```python
from build123d import *

# Parameters (mm, degrees)
F0_W        = 33.02
F0_H        = 101.6
F1_DEPTH    = 2.54
F2_W        = 33.02
F2_H        = 101.6
F2_W_2      = 5.08
F2_H_2      = 2.54
F3_DEPTH    = 19.05
F2_W_3      = 27.94
F2_H_3      = 27.94
F2_W_4      = 1.8288
F2_H_4      = 4.572
F4_DEPTH    = 2.54
F5_DEPTH    = 5.08
F7_W        = 3.1588217151
F7_H        = 3.175
F8_DEPTH    = 25.4
F9_T1_DEPTH = 2.54
F10_W       = 0.4572
F10_H       = 4.572
F10_W_2     = 1.8288
F10_W_3     = 2.286
F11_DEPTH   = 1.27
F13_DEPTH   = 6.35


# Not quite as in the source:
# - a fillet or chamfer that OpenCascade refuses, or shapes differently, is made with other operations: its cross-section is extruded or revolved along the edge and cut away or added


with BuildPart() as f1:
    # F0 (on Top) → F1 (new body)
    with BuildSketch(Plane.XY):
        with Locations((16.51, 50.8)):
            Rectangle(F0_W, F0_H)
    extrude(amount=F1_DEPTH)

    # F2 (on face) → F3 (join)
    with BuildSketch(Plane.XY.offset(2.54)):
        with Locations((16.51, 50.8)):
            Rectangle(F2_W, F2_H)
        Polygon((30.48, 2.54), (2.54, 2.54), (2.54, 64.77), (2.54, 67.31), (2.54, 71.12), (2.54, 99.06), (30.48, 99.06), (30.48, 71.12), (30.48, 67.31), (30.48, 64.77), align=None, mode=Mode.SUBTRACT)
        with Locations((5.08, 66.04)):
            Rectangle(F2_W_2, F2_H_2)
        with Locations((27.94, 66.04)):
            Rectangle(F2_W_2, F2_H_2)
    extrude(amount=F3_DEPTH)

    # F2 (on face) → F4 (join)
    with BuildSketch(Plane.XY.offset(2.54)):
        with Locations((16.51, 85.09)):
            Rectangle(F2_W_3, F2_H_3)
        with Locations((9.8806, 82.3468)):
            Rectangle(F2_W_4, F2_H_4, mode=Mode.SUBTRACT)
        with Locations((23.1394, 82.3468)):
            Rectangle(F2_W_4, F2_H_4, mode=Mode.SUBTRACT)
    extrude(amount=F4_DEPTH)

    # F2 (on face) → F5 (join)
    with BuildSketch(Plane.XY.offset(2.54)):
        with Locations((9.8806, 82.3468)):
            Rectangle(F2_W_4, F2_H_4)
        with Locations((23.1394, 82.3468)):
            Rectangle(F2_W_4, F2_H_4)
    extrude(amount=F5_DEPTH)

    # F7 (on face) → F8 (cut)
    with BuildSketch(Plane.XZ.offset(-99.06)):
        Polygon((10.795, 9.525), (10.795, 8.89), (24.0538, 8.89), (24.0538, 21.59), (10.795, 21.59), (10.795, 12.7), align=None)
        with Locations((9.2155891424, 11.1125)):
            Rectangle(F7_W, F7_H)
    extrude(amount=-F8_DEPTH, mode=Mode.SUBTRACT)

    # F9: fillet of radius 1.651 on 2 edges, made by hand

    # F9_s2 → F9_t1 (join)
    with BuildSketch(Plane.XZ.offset(-101.6)):
        with BuildLine():
            ThreePointArc((9.2871782849, 12.7), (8.1197449891, 12.2164332957), (7.6361782849, 11.049))
            Line((7.6361782849, 11.049), (7.6361782849, 12.7))
            Line((7.6361782849, 12.7), (9.2871782849, 12.7))
        make_face()
        with BuildLine():
            ThreePointArc((7.6361782849, 11.176), (8.1197449891, 10.0085667043), (9.2871782849, 9.525))
            Line((9.2871782849, 9.525), (7.6361782849, 9.525))
            Line((7.6361782849, 9.525), (7.6361782849, 11.176))
        make_face()
    extrude(amount=F9_T1_DEPTH)

    # F10 (on face) → F11 (join)
    with BuildSketch(Plane.XY.offset(7.62)):
        with Locations((11.0236, 82.3468)):
            Rectangle(F10_W, F10_H)
        with Locations((9.8806, 82.3468)):
            Rectangle(F10_W_2, F10_H)
        with Locations((22.9108, 82.3468)):
            Rectangle(F10_W_3, F10_H)
    extrude(amount=F11_DEPTH)

    # F12 (on face) → F13 (cut)
    with BuildSketch(Plane.XZ.offset(-80.0608)):
        Polygon((10.795, 8.89), (11.2522, 7.62), (11.2522, 8.89), align=None)
        Polygon((21.7678, 7.62), (22.225, 8.89), (21.7678, 8.89), align=None)
    extrude(amount=-F13_DEPTH, mode=Mode.SUBTRACT)


solid = f1.part
```
The model under review builds one solid part; all positions refer to its coordinate system, in mm. A direction names the side the tool comes from. Round coordinates to 2 decimals unless told otherwise and drop trailing zeros. Order: outer loops, then holes, each group sorted by start corner. A loop starts at its lowest first (then second) coordinate and runs counter-clockwise, first axis right, second up.
(1) Mouldability with a two-part tool opening along Z and no side actions: class faces 1 (the face through (8.13, 100.35, 10)), 2 (the face through (25.4, 66, 12)), 3 (the face through (17, 100, 8.89)) as released by +Z, released by -Z, zero draft, split by the parting line, or undercut.
Working result:
face 1: undercut
face 2: zero draft
face 3: released by +Z
(2) Wall thickness on L1, parallel to Y at x = 7, z = 15.75; L2, parallel to Y at x = 10, z = 8; L3, parallel to X at y = 31, z = 20.75: over which ranges is each line inside the solid? List them lowest first.
Working result:
L1: y = 0 to 2.54, 64.77 to 67.31, 99.06 to 101.6
L2: y = 0 to 2.54, 80.06 to 84.63, 99.06 to 101.6
L3: x = 0 to 2.54, 30.48 to 33.02
(3) Tool access review of faces 4 (the face through (8.155, 100.348, 12.251)), 5 (the face through (30.48, 83, 12)), 6 (the face through (24.054, 100, 15)): name each direction out of +Z, -Z, +X, -X, +Y, -Y from which nothing blocks a thin tool from reaching the whole face with its end or side.
Working result:
face 4: +Y
face 5: +Z
face 6: +Z, +Y
(4) Take a section at D-D, the plane x = 28.5. State the section outline as (y, z) points, plus the area to 3 significant figures.
Working result:
outline: (0, 0) - (101.6, 0) - (101.6, 21.59) - (99.06, 21.59) - (99.06, 5.08) - (71.12, 5.08) - (71.12, 2.54) - (67.31, 2.54) - (67.31, 21.59) - (64.77, 21.59) - (64.77, 2.54) - (2.54, 2.54) - (2.54, 21.59) - (0, 21.59) - close
area: 474 mm2
(5) Take a section at C-C, the plane x = 17.5. State the section outline as (y, z) points.
Working result:
outline: (0, 0) - (101.6, 0) - (101.6, 8.89) - (99.06, 8.89) - (99.06, 5.08) - (71.12, 5.08) - (71.12, 2.54) - (2.54, 2.54) - (2.54, 21.59) - (0, 21.59) - close
(6) For P1, Ø10, axis at x = 8, y = 58, coming from the +Z side; P2, Ø1.3, axis at x = 14, y = 100, coming from the +Z side, all flat-tipped, find the tip position at first contact; note any pin that passes through.
Working result:
P1: stops at z = 2.54
P2: stops at z = 8.89
(7) Take a section at B-B, the plane y = 25. State the section outline as (x, z) points.
Working result:
outline: (0, 0) - (33.02, 0) - (33.02, 21.59) - (30.48, 21.59) - (30.48, 2.54) - (2.54, 2.54) - (2.54, 21.59) - (0, 21.59) - close
(8) Take a section at A-A, the plane z = 15.25. State the section outline as (x, y) points (3 decimals), plus the area to 3 significant figures.
Working result:
outline: (0, 0) - (33.02, 0) - (33.02, 101.6) - (24.054, 101.6) - (24.054, 99.06) - (30.48, 99.06) - (30.48, 67.31) - (25.4, 67.31) - (25.4, 64.77) - (30.48, 64.77) - (30.48, 2.54) - (2.54, 2.54) - (2.54, 64.77) - (7.62, 64.77) - (7.62, 67.31) - (2.54, 67.31) - (2.54, 99.06) - (10.795, 99.06) - (10.795, 101.6) - (0, 101.6) - close
area: 650 mm2
